from build123d import *

# Parameters (mm, degrees)
SKETCH_2_R          = 4.5
CUT_EXTRUDE_1_DEPTH = 40
SKETCH_3_R          = 3
CUT_EXTRUDE_2_DEPTH = 5


with BuildPart() as part:
    # Эскиз1 → Повернуть-Тонкостенный1 (revolve)
    with BuildSketch(Plane.XY, mode=Mode.PRIVATE) as revolve_1_sk:
        Polygon((19, 0), (43, 0), (50, 21), (52.889577147, 23.332201276), (58.302767501, 25.953006302), (58.738533119, 25.052946123), (53.42847461, 22.482072549), (50.856038751, 20.405838593), (43.72075922, -1), (19, -1), align=None)
    revolve(revolve_1_sk.sketch.rotate(Axis((0, 0, 0), (0, -1, 0)), 90), axis=Axis((0, 0, 0), (0, -1, 0)))

    # Эскиз2 → Вытянуть1 (cut, symmetric)
    with BuildSketch(Plane(origin=(0, 0, 0), x_dir=(1, 0, 0), z_dir=(0, 1, 0))):
        with Locations(Location((30, 0, 0), (0, 0, 270))):
            Circle(SKETCH_2_R)
        with Locations(Location((-30, 0, 0), (0, 0, 270))):
            Circle(SKETCH_2_R)
        with Locations(Location((0, 30, 0), (0, 0, 270))):
            Circle(SKETCH_2_R)
        with Locations(Location((0, -30, 0), (0, 0, 270))):
            Circle(SKETCH_2_R)
    extrude(amount=CUT_EXTRUDE_1_DEPTH, both=True, mode=Mode.SUBTRACT)

    # Эскиз3 → Вытянуть2 (cut, symmetric)
    with BuildSketch(Plane(origin=(0, 0, 0), x_dir=(1, 0, 0), z_dir=(0, 1, 0))):
        with Locations(Location((20, -22.360679775, 0), (0, 0, 270))):
            Circle(SKETCH_3_R)
        with Locations(Location((-20, 22.360679775, 0), (0, 0, 270))):
            Circle(SKETCH_3_R)
    extrude(amount=CUT_EXTRUDE_2_DEPTH, both=True, mode=Mode.SUBTRACT)


solid = part.part
Part model, mm, in its own coordinate system. A direction names the side the tool comes from. Round coordinates to 2 decimals unless told otherwise and drop trailing zeros. Order: outer loops, then holes, each group sorted by start corner. A loop starts at its lowest first (then second) coordinate and runs counter-clockwise, first axis right, second up. Notation, with made-up numbers: (-5, 79.25) -> (47, 79.25) arc R13 ccw to (47, 84.25) -> close; hole circle Ø7 at (68, -15). An arc over 180 degrees is marked (long way). Put each result on its own line as item: value.
Q1. Pin check, flat tips, straight feed: pin 1 Ø4 at (x, y) = (-0.5, 5.5) entering from +Z; pin 2 Ø3 at (y, z) = (6, 23.5) entering from -X; pin 3 Ø8 at (x, y) = (-7, 9.5) entering from -Z. Stop position of each tip, or through.
From the geometry:
pin 1: stops at z = 46.55
pin 2: stops at x = -40.64
pin 3: stops at z = -48.15
Q2. Tool access for faces 1 (the face through (9, 0, -19)), 2 (the face through (18.85, -0.49, 25.13)): list every direction of +Z, -Z, +X, -X, +Y, -Y with a clear straight run to the whole face (end or side of a thin tool).
From the geometry:
face 1: +Y
face 2: +Y, -Y
Q3. Pull direction X, two halves, no side cores. Call faces 3 (the face through (44.52, 21.15, 23.16)), 4 (the face through (-16.1, 22.6, 51.2)), 5 (the face through (19, -1, 9)): pulls with the +X half, pulls with the -X half, needs draft (parallel to the pull), parting line crosses it, or undercut.
From the geometry:
face 3: undercut
face 4: parting line crosses it
face 5: needs draft
Q4. Band-saw the part on B-B (y = 11.5). Give the cut face in (x, z), and give its area (3 significant figures).
From the geometry:
outline: circle Ø95.77 at (0, 0); hole circle Ø93.67 at (0, 0)
area: 314 mm2
Q5. Wall check: line 1 (X direction, y = -0.2, z = 0); line 2 (X direction, y = 17, z = -29.5); line 3 (Z direction, x = -40, y = 4.75). Give the ranges that are in metal, low to high. Write a range as [from, to].
From the geometry:
line 1: x = [-43.99, -34.5], [-25.5, -19], [19, 25.5], [34.5, 43.99]
line 2: x = [-40.02, -38.71], [38.71, 40.02]
line 3: z = [-21.97, -19.69], [19.69, 21.97]
Q6. Band-saw the part on A-A (z = 0). Give the cut face in (x, y).
From the geometry:
outline: (-58.74, 25.05) -> (-53.43, 22.48) -> (-50.86, 20.41) -> (-43.72, -1) -> (-34.5, -1) -> (-34.5, 0) -> (-43, 0) -> (-50, 21) -> (-52.89, 23.33) -> (-58.3, 25.95) -> close; (-25.5, -1) -> (-19, -1) -> (-19, 0) -> (-25.5, 0) -> close; (19, -1) -> (25.5, -1) -> (25.5, 0) -> (19, 0) -> close; (34.5, -1) -> (43.72, -1) -> (50.86, 20.41) -> (53.43, 22.48) -> (58.74, 25.05) -> (58.3, 25.95) -> (52.89, 23.33) -> (50, 21) -> (43, 0) -> (34.5, 0) -> close
